from build123d import *

# Parameters (mm, degrees)
BOSS_EXTRUDE1_DEPTH = 45
BOSS_EXTRUDE2_START = 16
SKETCH1_3_R         = 4.5
SKETCH1_3_R_2       = 1.75
BOSS_EXTRUDE2_DEPTH = 13
CUT_EXTRUDE1_START  = 16
SKETCH5_R           = 5.5
CUT_EXTRUDE1_DEPTH  = 25
SKETCH6_R           = 2.6
CUT_EXTRUDE2_DEPTH  = 15
CUT_EXTRUDE4_START  = 49.4
SKETCH5_4_R         = 5.5
CUT_EXTRUDE4_DEPTH  = 20.4
FILLET1_R           = 0.5
FILLET2_R           = 5
SKETCH7_R           = 5.5
CUT_EXTRUDE3_DEPTH  = 3
SKETCH8_R           = 3.001117943
SKETCH8_R_2         = 3.734433125
BOSS_EXTRUDE5_DEPTH = 0.4
SKETCH9_W           = 2.236067978
SKETCH9_H           = 16
CUT_EXTRUDE5_DEPTH  = 10
FILLET4_R           = 5


with BuildPart() as part:
    # Sketch1 → Boss-Extrude1 (new body)
    with BuildSketch(Plane(origin=(0, 0, 0), x_dir=(1, 0, 0), z_dir=(0, 1, 0))):
        with BuildLine():
            Line((-46.5, 4.5), (-46.5, -2))
            Line((-46.5, -2), (-4.031128874, -2))
            ThreePointArc((-4.031128874, -2), (-3.824264635, 2.371708245), (0, 4.5))
            Line((0, 4.5), (-46.5, 4.5))
        make_face()
    extrude(amount=BOSS_EXTRUDE1_DEPTH)

    # Sketch1<3> → Boss-Extrude2 (add)
    # profile 1 of 2: a face of its own
    with BuildSketch(Plane(origin=(0, 0, 0), x_dir=(1, 0, 0), z_dir=(0, 1, 0)).offset(BOSS_EXTRUDE2_START)):
        Circle(SKETCH1_3_R)
        Polygon((-2.857883832, -1.65), (0, -3.3), (2.857883832, -1.65), (2.857883832, 1.65), (0, 3.3), (-2.857883832, 1.65), align=None, mode=Mode.SUBTRACT)
    # profile 2 of 2: a face of its own
    with BuildSketch(Plane(origin=(0, 0, 0), x_dir=(1, 0, 0), z_dir=(0, 1, 0)).offset(BOSS_EXTRUDE2_START)):
        Polygon((-2.857883832, 1.65), (-2.857883832, -1.65), (0, -3.3), (2.857883832, -1.65), (2.857883832, 1.65), (0, 3.3), align=None)
        with Locations(Location((0, 0, 0), (0, 0, 90))):
            Circle(SKETCH1_3_R_2, mode=Mode.SUBTRACT)
    extrude(amount=BOSS_EXTRUDE2_DEPTH)

    # Sketch5 → Cut-Extrude1 (cut)
    with BuildSketch(Plane(origin=(0, 0, 0), x_dir=(1, 0, 0), z_dir=(0, 1, 0)).offset(CUT_EXTRUDE1_START)):
        Circle(SKETCH5_R)
    extrude(amount=-CUT_EXTRUDE1_DEPTH, mode=Mode.SUBTRACT)

    # Sketch6 → Cut-Extrude2 (cut)
    with BuildSketch(Plane.XY.offset(2)):
        with Locations((-36.5, 36.417335992)):
            Circle(SKETCH6_R)
        with Locations((-36.5, 9.832941716)):
            Circle(SKETCH6_R)
    extrude(amount=-CUT_EXTRUDE2_DEPTH, mode=Mode.SUBTRACT)

    # Sketch5<4> → Cut-Extrude4 (cut)
    with BuildSketch(Plane(origin=(0, 0, 0), x_dir=(1, 0, 0), z_dir=(0, 1, 0)).offset(CUT_EXTRUDE4_START)):
        Circle(SKETCH5_4_R)
    extrude(amount=-CUT_EXTRUDE4_DEPTH, mode=Mode.SUBTRACT)

    # Fillet1
    fillet1_edges = [part.edges().sort_by_distance(p)[0] for p in [
        (-3.16227766, 8, -4.5),
    ]]
    fillet(fillet1_edges, radius=FILLET1_R)

    # Fillet2
    fillet2_edges = [part.edges().sort_by_distance(p)[0] for p in [
        (-46.5, 45, -1.25),
        (-46.5, 0, -1.25),
    ]]
    fillet(fillet2_edges, radius=FILLET2_R)

    # Sketch7 → Cut-Extrude3 (cut)
    with BuildSketch(Plane(origin=(0, 0, -4.5), x_dir=(-1, 0, 0), z_dir=(0, 0, -1))):
        with Locations((36.5, 36.417335992)):
            Circle(SKETCH7_R)
        with Locations((36.5, 9.832941716)):
            Circle(SKETCH7_R)
    extrude(amount=-CUT_EXTRUDE3_DEPTH, mode=Mode.SUBTRACT)

    # Sketch8 → Boss-Extrude5 (add)
    with BuildSketch(Plane(origin=(0, 0, -1.5), x_dir=(-1, 0, 0), z_dir=(0, 0, -1))):
        with Locations((36.5, 36.417335992)):
            Circle(SKETCH8_R)
        with Locations((36.5, 9.832941716)):
            Circle(SKETCH8_R_2)
    extrude(amount=-BOSS_EXTRUDE5_DEPTH)

    # Sketch9 → Cut-Extrude5 (cut)
    with BuildSketch(Plane(origin=(0, 0, -4.5), x_dir=(-1, 0, 0), z_dir=(0, 0, -1))):
        Polygon((5.5, 16), (4.472135955, 16), (4.472135955, 0), (21.5, 0), align=None)
        with Locations((3.354101966, 8)):
            Rectangle(SKETCH9_W, SKETCH9_H)
        Polygon((3.16227766, 29), (3.16227766, 45), (-0.050353192, 45), (-0.050353192, 29), (0, 29), align=None)
        Polygon((5.5, 29), (21.5, 45), (3.16227766, 45), (3.16227766, 29), align=None)
    extrude(amount=-CUT_EXTRUDE5_DEPTH, mode=Mode.SUBTRACT)

    # Fillet4
    # the kernel refuses this fillet: 5 mm, written as the material it adds along each edge
    with BuildSketch(Plane(origin=(-5.5, 29, 7.17766953), x_dir=(-0.7071067811865427, 0.7071067811865525, 0), z_dir=(0, 0, -1))) as fillet4_piece_1_section:
        with BuildLine():
            CenterArc((FILLET4_R * 0.414213562373, FILLET4_R), FILLET4_R, 225, 45)
            Line((-FILLET4_R * 0.292893218813, FILLET4_R * 0.292893218813), (0, 0))
            Line((0, 0), (FILLET4_R * 0.414213562373, 0))
        make_face()
    fillet4_piece_1 = extrude(amount=16.855339059, mode=Mode.PRIVATE)
    fillet4_piece_1 = fillet4_piece_1 & Plane(origin=(0, 29.007513744, 0), x_dir=(1, 0, 0), z_dir=(0, -1, 0)) * Cylinder(4.5, 42, mode=Mode.PRIVATE)
    add(fillet4_piece_1)
    with BuildSketch(Plane(origin=(-5.5, 29, 2), x_dir=(-0.7071067811865431, 0.7071067811865518, 0), z_dir=(0, 0, -1)), Plane(origin=(-5.5, 16, 2), x_dir=(1, 0, 0), z_dir=(0, 0, -1))) as fillet4_piece_2:
        with BuildLine():
            CenterArc((FILLET4_R * 0.414213562373, FILLET4_R), FILLET4_R, 225, 45)
            Line((-FILLET4_R * 0.292893218813, FILLET4_R * 0.292893218813), (0, 0))
            Line((0, 0), (FILLET4_R * 0.414213562373, 0))
        make_face()
    extrude(amount=6.5)
    with BuildSketch(Plane(origin=(-5.5, 16, 7.17766953), x_dir=(1, 0, 0), z_dir=(0, 0, -1))) as fillet4_piece_3_section:
        with BuildLine():
            CenterArc((FILLET4_R * 0.414213562373, FILLET4_R), FILLET4_R, 225, 45)
            Line((-FILLET4_R * 0.292893218813, FILLET4_R * 0.292893218813), (0, 0))
            Line((0, 0), (FILLET4_R * 0.414213562373, 0))
        make_face()
    fillet4_piece_3 = extrude(amount=16.855339059, mode=Mode.PRIVATE)
    fillet4_piece_3 = fillet4_piece_3 & Plane(origin=(0, 15.992486256, 0), x_dir=(1, 0, 0), z_dir=(0, -1, 0)) * Cylinder(4.5, 42, mode=Mode.PRIVATE)
    add(fillet4_piece_3)
    # the kernel refuses this fillet: 5 mm, written as the material it takes off along each edge
    with BuildSketch(Plane(origin=(-21.5, 0, -9.67766953), x_dir=(0.7071067811865441, 0.7071067811865509, 0), z_dir=(0, 0, 1)), Plane(origin=(-21.5, 45, -9.67766953), x_dir=(-1, 0, 0), z_dir=(0, 0, 1))) as fillet4_2_piece_1:
        with BuildLine():
            CenterArc((FILLET4_R * 0.414213562373, FILLET4_R), FILLET4_R, 225, 45)
            Line((-FILLET4_R * 0.292893218813, FILLET4_R * 0.292893218813), (0, 0))
            Line((0, 0), (FILLET4_R * 0.414213562373, 0))
        make_face()
    extrude(amount=16.855339059, mode=Mode.SUBTRACT)


solid = part.part
The listing builds one solid part. Answer for the finished solid, in the listing's coordinates (mm). A direction names the side the tool comes from. Coordinates: 2 decimals unless noted, no trailing zeros. Order: outer loops, then holes, each group sorted by start corner. A loop starts at its lowest first (then second) coordinate and runs counter-clockwise, first axis right, second up.
Q1. For a pull along Y with two mould halves and no side action, classify faces 6 (the face through (-38.416, 11.59, 0.472)), 7 (the face through (-21.68, 0.37, -1.3)), 8 (the face through (-21.63, 44.61, -1.3)) as pulls with the +Y half, pulls with the -Y half, needs draft (parallel to the pull), parting line crosses it, or undercut.
Q2. A cutting plane is placed at B-B, the plane y = 18.5. Write down the section's boundary in (x, z).
Q3. A cutting plane is placed at D-D, the plane y = 11. Write down the section's boundary in (x, z).
Q4. A cutting plane is placed at C-C, the plane x = -36.5. Write down the section's boundary in (y, z), and give its area (3 significant figures).
Q5. A cutting plane is placed at A-A, the plane z = 1. Write down the section's boundary in (x, y), and give its area (3 significant figures).
Q6. Which of the six approach directions +Z, -Z, +X, -X, +Y, -Y give full straight-line access (tool end or side, diameter ignored) to faces 1 (the face through (1, 29, -2)), 2 (the face through (-31.005, 36.659, -3.021)), 3 (the face through (0, 16, -2)), 4 (the face through (-36, 10, -1.1)), 5 (the face through (1.71, 22.41, 0.38))?
Q7. Consider line 1 (Y direction, x = -36.5, z = -3); line 2 (Y direction, x = -36.5, z = 1); line 3 (X direction, y = 22, z = 0). Determine where each line is inside the solid, lowest interval first.
Q8. Given P1, Ø8.5, axis at x = -36.5, y = 9.83, coming from the -Z side; P2, Ø1.6, axis at x = -35.5, y = 11, coming from the +Z side; P3, Ø1.5, axis at y = 5.5, z = 3, coming from the -X side; P4, Ø5.5, axis at x = -35.5, y = 35.5, coming from the +Z side, each flat-ended and moving along its own axis, determine where each tip first touches the part or whether it passes through.
Answers follow:
1. face 6: undercut
1. face 7: pulls with the -Y half
1. face 8: pulls with the +Y half
2. outline: (-46.5, -4.5) - (0, -4.5) arc R4.5 ccw (long way) to (-4.03, 2) - (-46.5, 2) - close; hole circle Ø3.5 at (0, 0)
3. outline: (-46.5, -4.5) - (-41.87, -4.5) - (-41.87, -1.5) - (-31.13, -1.5) - (-31.13, -4.5) - (-10.5, -4.5) - (-10.5, 2) - (-34.18, 2) - (-34.18, -1.1) - (-38.82, -1.1) - (-38.82, 2) - (-46.5, 2) - close
4. outline: (0, -4.5) - (4.33, -4.5) - (4.33, -1.5) - (15.33, -1.5) - (15.33, -4.5) - (30.92, -4.5) - (30.92, -1.5) - (41.92, -1.5) - (41.92, -4.5) - (45, -4.5) - (45, 2) - (39.02, 2) - (39.02, -1.1) - (33.82, -1.1) - (33.82, 2) - (12.43, 2) - (12.43, -1.1) - (7.23, -1.1) - (7.23, 2) - (0, 2) - close
4. area: 194 mm2
5. outline: (-46.5, 5) arc R5 ccw to (-41.5, 0) - (-23.57, 0) arc R5 ccw to (-20.04, 1.46) - (-6.96, 14.54) arc R5 cw to (-3.43, 16) - (-1.44, 16) - (-1.44, 29) - (-3.43, 29) arc R5 cw to (-6.96, 30.46) - (-20.04, 43.54) arc R5 ccw to (-23.57, 45) - (-41.5, 45) arc R5 ccw to (-46.5, 40) - close; (1.44, 16) - (4.39, 16) - (4.39, 29) - (1.44, 29) - close; hole circle Ø5.2 at (-36.5, 9.83); hole circle Ø5.2 at (-36.5, 36.42)
5. area: 1,630 mm2
6. face 1: +Z, -Z, +X, +Y
6. face 2: -Z
6. face 3: +Z, -Z, +X, -Y
6. face 4: +Z
6. face 5: +Y, -Y
7. line 1: y = 0 to 4.33, 15.33 to 30.92, 41.92 to 45
7. line 2: y = 0 to 7.23, 12.43 to 33.82, 39.02 to 45
7. line 3: x = -46.5 to -1.75, 1.75 to 4.5
8. P1: stops at z = -1.5
8. P2: stops at z = -1.1
8. P3: passes through
8. P4: stops at z = 2
